Verification items for the finished model (mm, model axes). A direction names the side the tool comes from. Give positions to 0.01 mm unless a question says otherwise; leave off trailing zeros. Order: outer loops, then holes, each group sorted by start corner. A loop starts at its lowest first (then second) coordinate and runs counter-clockwise, first axis right, second up. Notation, with made-up numbers: (86, 11) - (109, 11) arc R16 ccw to (109, 27) - close; hole circle Ø9 at (-32, 34). An arc over 180 degrees is marked (long way). Answer as a JSON object with one key per item and string values.
```python
from build123d import *

# Parameters (mm, degrees)
SKETCH1_W           = 5
SKETCH1_H           = 10
BOSS_EXTRUDE1_DEPTH = 10
FILLET3_R           = 1


with BuildPart() as part:
    # Sketch1 → Boss-Extrude1 (new body)
    with BuildSketch(Plane(origin=(0, 0, 0), x_dir=(1, 0, 0), z_dir=(0, 1, 0))):
        Polygon((142.399069508, 0.29194512), (-22.600930492, 0.29194512), (-22.600930492, 15.29194512), (-11.557039121, 15.29194512), (-11.557039121, 25.29194512), (-22.600930492, 25.29194512), (-32.600930492, 25.29194512), (-32.600930492, 12.072059565), (-32.600930492, 0.29194512), (-32.600930492, -9.70805488), (-14.486354187, -9.70805488), (12.890864677, -9.70805488), (152.399069508, -9.70805488), (152.399069508, 7.072059565), (152.399069508, 38.391958761), (152.399069508, 50.29194512), (142.399069508, 50.29194512), (127.399069508, 50.29194512), (127.399069508, 40.29194512), (142.399069508, 40.29194512), (142.399069508, 25.29194512), (142.399069508, 15.29194512), align=None)
        with Locations((139.899069508, 20.29194512)):
            Rectangle(SKETCH1_W, SKETCH1_H)
    extrude(amount=BOSS_EXTRUDE1_DEPTH)

    # Fillet3
    fillet3_edges = [part.edges().sort_by_distance(p)[0] for p in [
        (-11.557039121, 5, -15.29194512),
        (-22.600930492, 5, -15.29194512),
        (-22.600930492, 5, -0.29194512),
        (142.399069508, 5, -0.29194512),
        (142.399069508, 5, -15.29194512),
        (137.399069508, 5, -15.29194512),
        (137.399069508, 5, -25.29194512),
        (142.399069508, 5, -25.29194512),
        (142.399069508, 5, -40.29194512),
        (127.399069508, 5, -40.29194512),
    ]]
    fillet(fillet3_edges, radius=FILLET3_R)


solid = part.part
```
(1) Section check B-B (y = 2.25). Record the cut outline in (x, z).
Computed values:
{"outline": "(-32.6, -25.29) - (-11.56, -25.29) - (-11.56, -16.29) arc R1 ccw to (-12.56, -15.29) - (-21.6, -15.29) arc R1 cw to (-22.6, -14.29) - (-22.6, -1.29) arc R1 cw to (-21.6, -0.29) - (141.4, -0.29) arc R1 cw to (142.4, -1.29) - (142.4, -14.29) arc R1 cw to (141.4, -15.29) - (138.4, -15.29) arc R1 ccw to (137.4, -16.29) - (137.4, -24.29) arc R1 ccw to (138.4, -25.29) - (141.4, -25.29) arc R1 cw to (142.4, -26.29) - (142.4, -39.29) arc R1 cw to (141.4, -40.29) - (128.4, -40.29) arc R1 ccw to (127.4, -41.29) - (127.4, -50.29) - (152.4, -50.29) - (152.4, 9.71) - (-32.6, 9.71) - close"}
(2) Release check for a two-part mould opening along Z. For faces 1 (the flat face through (-22.601, 5, -8)), 2 (the flat face through (140, 5, -50.292)), 3 (the flat face through (66, 0, 2)) record: pulls with the +Z half, pulls with the -Z half, needs draft (parallel to the pull), parting line crosses it, or undercut.
Computed values:
{"face 1": "undercut", "face 2": "pulls with the -Z half", "face 3": "needs draft"}
(3) Section check C-C (z = -44). Record the cut outline in (x, y).
Computed values:
{"outline": "(127.4, 0) - (152.4, 0) - (152.4, 10) - (127.4, 10) - close"}
(4) Section check D-D (x = 117.5). Record the cut outline in (y, z), then the cut area to 3 significant figures.
Computed values:
{"outline": "(0, -0.29) - (10, -0.29) - (10, 9.71) - (0, 9.71) - close", "area": "100 mm²"}
(5) Material ranges on line 1 along X through (y, z) = (6.5, -16.5); line 2 along X through (y, z) = (4.5, -12); line 3 along Z through (x, y) = (130, 4.5), recorded low to high. Write a range as [from, to].
Computed values:
{"line 1": "x = [-32.6, -11.56], [137.4, 152.4]", "line 2": "x = [-32.6, -22.6], [142.4, 152.4]", "line 3": "z = [-50.29, -40.29], [-0.29, 9.71]"}
(6) Access from +Z, -Z, +X, -X, +Y, -Y to the whole of each face (thin tool, end or side, straight path). Record for faces 4 (the flat face through (140, 5, -25.292)), 5 (the flat face through (-22, 5, -25.292)), 6 (the flat face through (-11.557, 5, -21)), 7 (the flat face through (140, 5, -15.292)), 8 (the flat face through (59, 5, 9.708)).
Computed values:
{"face 4": "-X, +Y, -Y", "face 5": "-Z, -X, +Y, -Y", "face 6": "-Z, +Y, -Y", "face 7": "+Y, -Y", "face 8": "+Z, +X, -X, +Y, -Y"}
(7) Section check A-A (z = -22). Record the cut outline in (x, y), then the cut area to 3 significant figures.
Computed values:
{"outline": "(-32.6, 0) - (-11.56, 0) - (-11.56, 10) - (-32.6, 10) - close; (137.4, 0) - (152.4, 0) - (152.4, 10) - (137.4, 10) - close", "area": "360 mm²"}
(8) Gauge pin test, flat ends, axial feed: pin 1 Ø5 at (y, z) = (3, -34.5) entering from -X; pin 2 Ø3 at (x, y) = (80, 6) entering from -Z; pin 3 Ø5 at (x, z) = (133, -19) entering from +Y. Record the tip position at first contact, or that the pin passes through.
Computed values:
{"pin 1": "stops at x = 142.4", "pin 2": "stops at z = -0.29", "pin 3": "passes through"}
